```python
from build123d import *

# Parameters (mm, degrees)
BOSS_EXTRUDE1_DEPTH = 304.8
CUT_EXTRUDE1_DEPTH  = 313.185013253


with BuildPart() as part:
    # Sketch1 → Boss-Extrude1 (new body)
    with BuildSketch(Plane(origin=(0, 0, 0), x_dir=(0, 0, -1), z_dir=(1, 0, 0))):
        Polygon((0, 0), (50.8, 0), (50.8, 6.35), (6.35, 6.35), (6.35, 50.8), (0, 50.8), align=None)
    extrude(amount=BOSS_EXTRUDE1_DEPTH)

    # Sketch2 → Cut-Extrude1 (cut, through all)
    with BuildSketch(Plane(origin=(0, 6.35, 0), x_dir=(1, 0, 0), z_dir=(0, 1, 0))):
        with BuildLine():
            Line((53.975, 42.8625), (53.975, 17.4625))
            ThreePointArc((53.975, 17.4625), (50.8, 14.2875), (47.625, 17.4625))
            Line((47.625, 17.4625), (47.625, 42.8625))
            ThreePointArc((47.625, 42.8625), (50.8, 46.0375), (53.975, 42.8625))
        make_face()
        with BuildLine():
            Line((250.825, 42.8625), (250.825, 17.4625))
            ThreePointArc((250.825, 17.4625), (254, 14.2875), (257.175, 17.4625))
            Line((257.175, 17.4625), (257.175, 42.8625))
            ThreePointArc((257.175, 42.8625), (254, 46.0375), (250.825, 42.8625))
        make_face()
    extrude(amount=-CUT_EXTRUDE1_DEPTH, mode=Mode.SUBTRACT)


solid = part.part
```
CAD build for the part. Positions are in the model's coordinates, mm. A direction names the side the tool comes from. Round coordinates to 2 decimals unless told otherwise and drop trailing zeros. Order: outer loops, then holes, each group sorted by start corner. A loop starts at its lowest first (then second) coordinate and runs counter-clockwise, first axis right, second up. Notation, with made-up numbers: (37, -25) - (84, -25) arc R19 cw to (84, -19) - close; hole circle Ø9 at (86, 53). An arc over 180 degrees is marked (long way). Use CSV: the item, a comma, the result in double quotes. Start each with the question number.
1) Tool access for faces 1 (the flat face through (150, 50.8, -3)), 2 (the cylindrical face through (50.87, 3.22, -14.29)), 3 (the flat face through (150, 6.35, -29)): list every direction of +Z, -Z, +X, -X, +Y, -Y with a clear straight run to the whole face (end or side of a thin tool).
2) Saw through at C-C (x = 95). List the corners of the cut face in (y, z).
3) Saw through at A-A (z = -25.5). List the corners of the cut face in (x, y) (3 decimals).
4) Saw through at D-D (y = 36). List the corners of the cut face in (x, z), and give its area (3 significant figures).
5) Two-plate mould, pull along Z, no slides. Class faces 4 (the flat face through (257.175, 3, -30)), 5 (the flat face through (150, 3, -50.8)), 6 (the flat face through (304.8, 5, -14)): pulls with the +Z half, pulls with the -Z half, needs draft (parallel to the pull), parting line crosses it, or undercut.
6) Pin check, flat tips, straight feed: pin 1 Ø3 at (y, z) = (3.5, -33.5) entering from -X; pin 2 Ø6 at (x, z) = (86.5, -11) entering from +Y; pin 3 Ø2 at (x, y) = (83, 22) entering from -Z. Stop position of each tip, or through.
7) Wall check: L1, parallel to X at y = 3, z = -40.5 (3 decimals); L2, parallel to Y at x = 99.5, z = -21; L3, parallel to Z at x = 143, y = 48. Give the ranges that are in metal, low to high. Write a range as [from, to].
8) Saw through at B-B (x = 50.8). List the corners of the cut face in (y, z), and give its area (3 significant figures).
Values follow:
1,face 1,"+Z, -Z, +X, -X, +Y"
1,face 2,"+Y, -Y"
1,face 3,"-Z, +X, -X, +Y"
2,outline,"(0, -50.8) - (6.35, -50.8) - (6.35, -6.35) - (50.8, -6.35) - (50.8, 0) - (0, 0) - close"
3,outline,"(0, 0) - (47.625, 0) - (47.625, 6.35) - (0, 6.35) - close; (53.975, 0) - (250.825, 0) - (250.825, 6.35) - (53.975, 6.35) - close; (257.175, 0) - (304.8, 0) - (304.8, 6.35) - (257.175, 6.35) - close"
4,outline,"(0, -6.35) - (304.8, -6.35) - (304.8, 0) - (0, 0) - close"
4,area,"1,940 mm2"
5,face 4,"undercut"
5,face 5,"pulls with the -Z half"
5,face 6,"needs draft"
6,pin 1,"stops at x = 0"
6,pin 2,"stops at y = 6.35"
6,pin 3,"stops at z = -6.35"
7,L1,"x = [0, 47.625], [53.975, 250.825], [257.175, 304.8]"
7,L2,"y = [0, 6.35]"
7,L3,"z = [-6.35, 0]"
8,outline,"(0, -50.8) - (6.35, -50.8) - (6.35, -46.04) - (0, -46.04) - close; (0, -14.29) - (6.35, -14.29) - (6.35, -6.35) - (50.8, -6.35) - (50.8, 0) - (0, 0) - close"
8,area,"403 mm2"
